```python
from build123d import *

# Parameters (mm, degrees)
F1_DEPTH     = 30.3
F2_R         = 1.6899494937
F3_W         = 26.949964059
F3_H         = 12.8249995296
F4_DEPTH     = 0.5
F5_R         = 0.2414213562
F6_W         = 1.2325234711
F6_H         = 1.1400654912
F6_W_2       = 1.3488382101
F6_H_2       = 1.1522620916
F6_W_3       = 1.4076605439
F6_W_4       = 1.4072209597
F6_W_5       = 1.4375131577
F6_W_6       = 1.4656018466
F6_W_7       = 1.4457069337
F6_W_8       = 1.4214487746
F6_W_9       = 1.4211460948
F6_W_10      = 1.4119520783
F6_W_11      = 1.4170180075
F6_W_12      = 1.4084377326
F6_W_13      = 1.4295475557
F7_DEPTH     = 0.5
F8_W         = 9.2926481739
F8_H         = 6.1567388475
F9_DEPTH     = 0.19
F10_T1_DEPTH = 11.7376448309
F10_T3_DEPTH = 6.1567388475
F10_T5_DEPTH = 6.1567388475


# Not quite as in the source:
# - a fillet or chamfer that OpenCascade refuses, or shapes differently, is made with other operations: its cross-section is extruded or revolved along the edge and cut away or added


with BuildPart() as f1:
    # F0 (on Right) → F1 (new body)
    with BuildSketch(Plane.YZ):
        Polygon((-44.1633068031, 1.9997905069), (-44.1343598068, 0), (-22.1343598068, 0), (-22.1343598068, 1), align=None)
    extrude(amount=F1_DEPTH)

    # F2
    f2_edges = [f1.edges().sort_by_distance(p)[0] for p in [
        (0, -22.13436, 0.5),
        (30.3, -22.13436, 0.5),
        (30.3, -44.148833, 0.999895),
        (0, -44.148833, 0.999895),
    ]]
    fillet(f2_edges, radius=F2_R)

    # F3 (on face) → F4 (cut)
    with BuildSketch(Plane(origin=(0, -0.0002071974, -0.0045652959), x_dir=(1, 0, 0), z_dir=(0, 0.0453386355, 0.9989716753))):
        with Locations((15.1350684769, -36.10308207)):
            Rectangle(F3_W, F3_H)
    extrude(amount=-F4_DEPTH, mode=Mode.SUBTRACT)

    # F5
    f5_edges = [f1.edges().sort_by_distance(p)[0] for p in [
        (1.660086, -42.483404, 1.67329),
        (28.610051, -42.483404, 1.67329),
        (15.135068, -42.472069, 1.923033),
        (15.135068, -42.494739, 1.423547),
        (1.660086, -36.066164, 1.632299),
        (1.660086, -29.671593, 1.091822),
        (1.660086, -36.088833, 1.132813),
        (28.610051, -29.671593, 1.091822),
        (15.135068, -29.660258, 1.341565),
        (15.135068, -29.682927, 0.842079),
        (28.610051, -36.066164, 1.632299),
        (28.610051, -36.088833, 1.132813),
    ]]
    fillet(f5_edges, radius=F5_R)

    # F6 (on face) → F7 (join)
    with BuildSketch(Plane(origin=(0, -0.0228765151, -0.5040511335), x_dir=(1, 0, 0), z_dir=(0, 0.0453386355, 0.9989716753))):
        with Locations((27.318617329, -41.3098782301)):
            Rectangle(F6_W, F6_H)
        with Locations((25.6510563195, -41.3037799299)):
            Rectangle(F6_W_2, F6_H_2)
        with Locations((23.7977188081, -41.3037799299)):
            Rectangle(F6_W_3, F6_H_2)
        with Locations((21.7823982239, -41.3037799299)):
            Rectangle(F6_W_4, F6_H_2)
        with Locations((19.8403866962, -41.3037799299)):
            Rectangle(F6_W_5, F6_H_2)
        with Locations((17.95785781, -41.3037799299)):
            Rectangle(F6_W_6, F6_H_2)
        with Locations((16.0227976739, -41.3037799299)):
            Rectangle(F6_W_7, F6_H_2)
        with Locations((13.9798414893, -41.3037799299)):
            Rectangle(F6_W_8, F6_H_2)
        with Locations((11.8983006105, -41.3037799299)):
            Rectangle(F6_W_9, F6_H_2)
        with Locations((9.9623361602, -41.3037799299)):
            Rectangle(F6_W_10, F6_H_2)
        with Locations((8.0330308992, -41.3037799299)):
            Rectangle(F6_W_11, F6_H_2)
        with Locations((6.0811268631, -41.3037799299)):
            Rectangle(F6_W_12, F6_H_2)
        with Locations((4.1761151515, -41.3037799299)):
            Rectangle(F6_W_13, F6_H_2)
    extrude(amount=F7_DEPTH)

    # F8 (on face) → F9 (cut)
    with BuildSketch(Plane(origin=(0, -0.0002071974, -0.0045652959), x_dir=(1, 0, 0), z_dir=(0, 0.0453386355, 0.9989716753))):
        with Locations((15.4813206755, -25.8142389357)):
            Rectangle(F8_W, F8_H)
    extrude(amount=-F9_DEPTH, mode=Mode.SUBTRACT)

    # F10: fillet of radius 0.7242640687 on 4 edges, made by hand

    # F10_s2 → F10_t1 (join)
    with BuildSketch(Plane.YZ.offset(9.61249826)):
        with BuildLine():
            ThreePointArc((-28.8631045752, 1.3053861423), (-28.6430306792, 1.1544220499), (-28.3832224346, 1.0934109616))
            Line((-28.3832224346, 1.0934109616), (-28.8717189159, 1.115581524))
            Line((-28.8717189159, 1.115581524), (-28.8631045752, 1.3053861423))
        make_face()
        with BuildLine():
            ThreePointArc((-22.7126968541, 1.026248004), (-22.945540921, 0.8958397321), (-23.2098076761, 0.8586139482))
            Line((-23.2098076761, 0.8586139482), (-22.7213111948, 0.8364433857))
            Line((-22.7213111948, 0.8364433857), (-22.7126968541, 1.026248004))
        make_face()
    extrude(amount=F10_T1_DEPTH)

    # F10_s4 → F10_t3 (join)
    with BuildSketch(Plane(origin=(0, -22.7124896567, 1.0308132999), x_dir=(1, 0, 0), z_dir=(0, -0.9989716753, 0.0453386355))):
        with BuildLine():
            ThreePointArc((10.8349965885, -0.0045699953), (11.061688683, -0.1454009974), (11.3239959199, -0.1945699953))
            Line((11.3239959199, -0.1945699953), (10.8349965885, -0.1945699953))
            Line((10.8349965885, -0.1945699953), (10.8349965885, -0.0045699953))
        make_face()
    extrude(amount=F10_T3_DEPTH)

    # F10_s6 → F10_t5 (join)
    with BuildSketch(Plane(origin=(0, -28.8628973778, 1.3099514382), x_dir=(1, 0, 0), z_dir=(0, 0.9989716753, -0.0453386355))):
        with BuildLine():
            ThreePointArc((20.1276447624, 0.0045699953), (19.9009526679, 0.1454009974), (19.638645431, 0.1945699953))
            Line((19.638645431, 0.1945699953), (20.1276447624, 0.1945699953))
            Line((20.1276447624, 0.1945699953), (20.1276447624, 0.0045699953))
        make_face()
    extrude(amount=F10_T5_DEPTH)


solid = f1.part
```
Could you check a few things on this model? Use its own coordinates, in mm. A direction names the side the tool comes from. Round coordinates to 2 decimals unless told otherwise and drop trailing zeros. Answer as CSV lines item,"result".
1) For pin 1 Ø1.5 at (x, y) = (10.5, -38.5) entering from -Z; pin 2 Ø1 at (x, y) = (25.5, -26.5) entering from +Z, each with a flat end and sliding along its axis, tell me the tip position at first contact or that it passes through.
From the geometry:
pin 1,"z = 0"
pin 2,"z = 1.22"
2) We'd pull the mould along X, two halves only. Please class faces 4 (the cylindrical face through (1, -44, 1)), 5 (the flat face through (27.31, -41.26, 1.87)), 6 (the cylindrical face through (1.587, -35.983, 1.56)): released by +X, released by -X, zero draft, split by the parting line, or undercut.
From the geometry:
face 4,"released by -X"
face 5,"zero draft"
face 6,"undercut"
3) If I drill on probe 1 along X at (y, z) = (-34.75, 1.3); probe 2 along Z at (x, y) = (29, -24.75); probe 3 along Z at (x, y) = (22, -30), over which ranges is the centre line in solid material (lowest first)?
From the geometry:
probe 1,"0 to 1.66, 28.61 to 30.3"
probe 2,"0 to 1.12"
probe 3,"0 to 0.86"
4) Which directions (+Z, -Z, +X, -X, +Y, -Y) give clear straight access to the entire face, cutting with the end or side of a thin tool? Please do faces 1 (the cylindrical face through (28.683, -35.983, 1.56)), 2 (the cylindrical face through (0.508, -22.616, 0.546)), 3 (the cylindrical face through (29.79, -43.67, 0.98)).
From the geometry:
face 1,"+Z"
face 2,"+Z, -Z, -X, +Y"
face 3,"-Z, +X, -Y"
